Work out the finished part from the listing and answer in its coordinate system (mm). Coordinates: 2 decimals unless noted, no trailing zeros. Loops run counter-clockwise (first coordinate to the right, second up) from the corner with the lowest first, then second, coordinate; pieces in that order, holes last. Notation, with made-up numbers: (-1.75, 80) -> (31.25, 80) arc R20 ccw to (31.25, 103) -> close; hole circle Ø11 at (57.25, 35.25). An arc over 180 degrees is marked (long way). Use a Markdown table: item, result. Add a question column.
```python
from build123d import *

# Parameters (mm, degrees)
SKETCH1_W           = 249.6
SKETCH1_H           = 150
BOSS_EXTRUDE1_DEPTH = 3
SKETCH2_R           = 20
CUT_EXTRUDE1_DEPTH  = 4
SKETCH3_W           = 40
SKETCH3_H           = 30
CUT_EXTRUDE2_DEPTH  = 5
SKETCH4_R           = 2.1
SKETCH4_R_2         = 4
CUT_EXTRUDE3_DEPTH  = 4


with BuildPart() as part:
    # Sketch1 → Boss-Extrude1 (new body)
    with BuildSketch(Plane.XY):
        with Locations((124.8, -75)):
            Rectangle(SKETCH1_W, SKETCH1_H)
    extrude(amount=BOSS_EXTRUDE1_DEPTH)

    # Sketch2 → Cut-Extrude1 (cut, through all)
    with BuildSketch(Plane.XY.offset(3)):
        with Locations((67.5, -67.5)):
            Circle(SKETCH2_R)
    extrude(amount=-CUT_EXTRUDE1_DEPTH, mode=Mode.SUBTRACT)

    # Sketch3 → Cut-Extrude2 (cut)
    with BuildSketch(Plane.XY.offset(3)):
        with Locations((229.6, -51)):
            Rectangle(SKETCH3_W, SKETCH3_H)
    extrude(amount=-CUT_EXTRUDE2_DEPTH, mode=Mode.SUBTRACT)

    # Sketch4 → Cut-Extrude3 (cut, through all)
    with BuildSketch(Plane.XY.offset(3)):
        with Locations((200.8, -5.5)):
            Circle(SKETCH4_R)
        with Locations((218.3, -5.5)):
            Circle(SKETCH4_R)
        with Locations((205.8, -18)):
            Circle(SKETCH4_R_2)
        with Locations((200.8, -30.5)):
            Circle(SKETCH4_R)
        with Locations((218.3, -30.5)):
            Circle(SKETCH4_R)
        with Locations((243.3, -5.5)):
            Circle(SKETCH4_R)
        with Locations((243.3, -30.5)):
            Circle(SKETCH4_R)
        with Locations((230.8, -18)):
            Circle(SKETCH4_R_2)
    extrude(amount=-CUT_EXTRUDE3_DEPTH, mode=Mode.SUBTRACT)


solid = part.part
```
Item 1: Section A-A (x = 67.5) is taken. Determine the outline of the cut face in (y, z), then the cut area to 3 significant figures.
Item 2: Section D-D (z = 1.95) is taken. Count the separate pieces of the cut face and the enclosed holes in it, then the cut area to 3 significant figures.
Item 3: Section B-B (x = 230.8) is taken. Determine the outline of the cut face in (y, z), then the cut area to 3 significant figures.
Item 4: Find the intervals of material crossed by probe 1 along Y at (x, z) = (200.8, 1.8); probe 2 along Y at (x, z) = (243.3, 1.3); probe 3 along X at (y, z) = (-66.5, 1.85), in increasing order.
Item 5: For a pull along Y with two mould halves and no side action, classify faces 1 (the face through (123, -74, 0)), 2 (the face through (234.615, -16.799, 1.521)) as +Y half, -Y half, draft (parallel to the pull), parting line (faces both ways), or undercut.
Item 6: Section C-C (y = -61) is taken. Determine the outline of the cut face in (x, z).
Item 7: Given pin 1 (5.5 mm diameter, centred on x = 200.8, y = -5.5, fed in from -Z), flat-ended and moving along its own axis, determine where the tip first touches the part or whether it passes through.
Output:
| question | item | result |
|---|---|---|
| 1 | outline | (-150, 0) -> (-87.5, 0) -> (-87.5, 3) -> (-150, 3) -> close; (-47.5, 0) -> (0, 0) -> (0, 3) -> (-47.5, 3) -> close |
| 1 | area | 330 mm2 |
| 2 | separate pieces | 1 |
| 2 | enclosed holes | 9 |
| 2 | area | 34,800 mm2 |
| 3 | outline | (-150, 0) -> (-66, 0) -> (-66, 3) -> (-150, 3) -> close; (-36, 0) -> (-22, 0) -> (-22, 3) -> (-36, 3) -> close; (-14, 0) -> (0, 0) -> (0, 3) -> (-14, 3) -> close |
| 3 | area | 336 mm2 |
| 4 | probe 1 | y = -150 to -32.6, -28.4 to -7.6, -3.4 to 0 |
| 4 | probe 2 | y = -150 to -66, -36 to -32.6, -28.4 to -7.6, -3.4 to 0 |
| 4 | probe 3 | x = 0 to 47.53, 87.47 to 249.6 |
| 5 | face 1 | draft |
| 5 | face 2 | undercut |
| 6 | outline | (0, 0) -> (48.59, 0) -> (48.59, 3) -> (0, 3) -> close; (86.41, 0) -> (209.6, 0) -> (209.6, 3) -> (86.41, 3) -> close |
| 7 | pin 1 | stops at z = 0 |
